```python
from build123d import *

# Parameters (mm, degrees)
F1_DEPTH = 3
F3_D     = 3.7973
F4_W     = 3
F4_H     = 5.08
F4_W_2   = 35
F4_H_2   = 8
F4_W_3   = 6.35
F4_H_3   = 3
F4_H_4   = 12.7
F4_W_4   = 12.7
F5_DEPTH = 3.001
F6_R     = 5.08


with BuildPart() as f1:
    # F0 (on Top) → F1 (new body)
    with BuildSketch(Plane.XY):
        Polygon((50.8, 41.275), (-50.8, 41.275), (-50.8, -6.985), (-60.96, -6.985), (-60.96, -41.275), (-30.4179767442, -75.565), (15.6730507807, -75.565), (15.6730507807, -76.835), (-29.2867906977, -76.835), (-23.6308604651, -83.185), (11.0115253904, -83.185), (11.0115253904, -84.455), (-22.4996744186, -84.455), (-15, -92.875), (-15, -142.875), (15, -142.875), (15, -92.875), (19.1061162791, -88.265), (-11.0115253904, -88.265), (-11.0115253904, -86.995), (20.2373023256, -86.995), (25.8932325581, -80.645), (-15.6730507807, -80.645), (-15.6730507807, -79.375), (27.0244186047, -79.375), (60.96, -41.275), (60.96, -6.985), (50.8, -6.985), align=None)
        Polygon((-15.6730507807, -73.025), (-43.9527019435, -41.275), (-6.35, -41.275), (-6.35, -73.025), align=None, mode=Mode.SUBTRACT)
        Polygon((6.35, -41.275), (43.9527019435, -41.275), (15.6730507807, -73.025), (6.35, -73.025), align=None, mode=Mode.SUBTRACT)
    extrude(amount=F1_DEPTH)

    # F3 (through all)
    with Locations(Plane.XY.offset(3)):
        with Locations((-59.46, -24.13), (59.46, -24.13)):
            Hole(F3_D / 2)

    # F4 (on face) → F5 (cut, through all)
    with BuildSketch(Plane.XY.offset(3)):
        with Locations((-59.46, -31.75)):
            Rectangle(F4_W, F4_H)
        with Locations((-59.46, -16.51)):
            Rectangle(F4_W, F4_H)
        with Locations((59.46, -16.51)):
            Rectangle(F4_W, F4_H)
        with Locations((59.46, -31.75)):
            Rectangle(F4_W, F4_H)
        with Locations((-33.3, 37.275)):
            Rectangle(F4_W_2, F4_H_2)
        with Locations((33.3, 37.275)):
            Rectangle(F4_W_2, F4_H_2)
        with Locations((-33.3, 25.425)):
            Rectangle(F4_W_3, F4_H_3)
        with Locations((33.3, 25.425)):
            Rectangle(F4_W_3, F4_H_3)
        with Locations((41.5, -5.925)):
            Rectangle(F4_W, F4_H_4)
        with Locations((-41.5, -5.925)):
            Rectangle(F4_W, F4_H_4)
        with Locations((0, -137.795)):
            Rectangle(F4_W_4, F4_H_3)
    extrude(amount=-F5_DEPTH, mode=Mode.SUBTRACT)

    # F6
    f6_edges = [f1.edges().sort_by_distance(p)[0] for p in [
        (-43.952702, -41.275, 1.5),
        (-6.35, -41.275, 1.5),
        (43.952702, -41.275, 1.5),
        (6.35, -41.275, 1.5),
        (15.673051, -73.025, 1.5),
        (-15.673051, -73.025, 1.5),
        (-6.35, -73.025, 1.5),
        (6.35, -73.025, 1.5),
    ]]
    fillet(f6_edges, radius=F6_R)


solid = f1.part
```
CAD build for the part. Positions are in the model's coordinates, mm. A direction names the side the tool comes from. Coordinates: 2 decimals unless noted, no trailing zeros. Write each loop counter-clockwise with the first axis right and the second up, starting at its lowest first coordinate (ties: lowest second). Pieces come first, ordered by that corner, then holes. Notation, with made-up numbers: (-24, 78) -> (7, 78) arc R14 ccw to (7, 90) -> close; hole circle Ø9 at (-10.5, 71.5). An arc over 180 degrees is marked (long way). Return JSON: item names as keys, results as strings. Group by question number.
Q1. Drill centre lines: line 1 (Y direction, x = -59.46, z = 0.6) (3 decimals); line 2 (Y direction, x = -5.5, z = 1.15) (3 decimals); line 3 (X direction, y = -43, z = 1.8). Where is each one in solid material? Low to high.
Q2. Which spindle directions (+Z, -Z, +X, -X, +Y, -Y) get a long thin tool onto all of the face, cutting with end or side? Do faces 1 (the face through (-7.9, -71.6, 1.5)), 2 (the face through (-1, -29, 0)). Say none if no direction does.
Q3. Pull direction Y, two halves, no side cores. Call faces 3 (the face through (43.755, -60.592, 1.479)), 4 (the face through (-1, -29, 3)), 5 (the face through (-37.293, -44.351, 1.521)): released by +Y, released by -Y, zero draft, split by the parting line, or undercut.
Q4. Cut at D-D, the plane x = 45. Give the cut face in (y, z) (3 decimals).
Q5. Flat gauge pins, fed straight in: pin 1 (1 mm diameter, centred on y = -80, z = 1.5, fed in from +X); pin 2 (1.5 mm diameter, centred on x = -60, z = 1.5, fed in from -Y); pin 3 (1.5 mm diameter, centred on x = -32, z = 2, fed in from +Y) (3 decimals). Where does each tip first touch, or does it go through?
Q6. Cut at B-B, the plane z = 1.75. State how many separate pieces and enclosed holes the cut face has, then the cut area to 3 significant figures.
Q7. Cut at A-A, the plane x = -26.5. Give the cut face in (y, z) (3 decimals), then the cut area to 3 significant figures.
Q8. Cut at C-C, the plane y = 13. Give the cut face in (x, z).
Returned:
{
 "1": {"line 1": "y = -42.959 to -34.29, -29.21 to -26.029, -22.231 to -19.05, -13.97 to -6.985", "line 2": "y = -142.875 to -139.295, -136.295 to -88.265, -86.995 to -84.455, -83.185 to -80.645, -79.375 to -76.835, -75.565 to 41.275", "line 3": "x = -59.42 to -36.44, -7.62 to 7.62, 36.44 to 59.42"},
 "2": {"face 1": "+Z, -Z", "face 2": "-Z, +X, -X, +Y, -Y"},
 "3": {"face 3": "released by -Y", "face 4": "zero draft", "face 5": "undercut"},
 "4": {"outline": "(-59.194, 0) -> (33.275, 0) -> (33.275, 3) -> (-59.194, 3) -> close"},
 "5": {"pin 1": "stops at x = -15.67", "pin 2": "stops at y = -43.19", "pin 3": "stops at y = 33.275"},
 "6": {"separate pieces": "1", "enclosed holes": "7", "area": "12,100 mm2"},
 "7": {"outline": "(-79.964, 0) -> (-76.835, 0) -> (-76.835, 3) -> (-79.964, 3) -> close; (-75.565, 0) -> (-60.869, 0) -> (-60.869, 3) -> (-75.565, 3) -> close; (-41.275, 0) -> (33.275, 0) -> (33.275, 3) -> (-41.275, 3) -> close", "area": "277 mm2"},
 "8": {"outline": "(-50.8, 0) -> (50.8, 0) -> (50.8, 3) -> (-50.8, 3) -> close"}
}
